Here's how the part is built. I have some questions about the finished solid (model axes, mm). A direction names the side the tool comes from. Give positions to 0.01 mm unless a question says otherwise; leave off trailing zeros. Write each loop counter-clockwise with the first axis right and the second up, starting at its lowest first coordinate (ties: lowest second). Pieces come first, ordered by that corner, then holes. Notation, with made-up numbers: (30, 50) - (51, 50) arc R22 cw to (51, 77) - close; hole circle Ø5 at (-21.75, 6). An arc over 180 degrees is marked (long way). Write each question's results on one line, items separated by ' | '. Start each with the question number.
Item 1: Will these pins go through, and if not, where does the flat tip stop? P1, Ø2.5, axis at x = -14, z = -15.5, coming from the -Y side; P2, Ø5.5, axis at x = 15, z = -16.5, coming from the -Y side; P3, Ø1.5, axis at x = 27, y = 1.5, coming from the +Z side; P4, Ø1.4, axis at x = 13.716, z = -13.716, coming from the +Y side.
Item 2: Suppose I cut it at A-A on x = 7.5. List the corners of the cut face in (y, z) for me.
Item 3: Suppose I cut it at B-B on y = 3.5. List the corners of the cut face in (x, z) for me (3 decimals), then the cut area to 3 significant figures.
Item 4: Suppose I cut it at D-D on x = -32. List the corners of the cut face in (y, z) for me, then the cut area to 3 significant figures.
Item 5: Which directions (+Z, -Z, +X, -X, +Y, -Y) give clear straight access to the entire face, cutting with the end or side of a thin tool? Please do faces 1 (the flat face through (19.05, 3, 25)), 2 (the flat face through (-11.43, 3, -14)), 3 (the flat face through (15, 0.508, -14)).
Item 6: Suppose I cut it at C-C on z = 22. List the corners of the cut face in (x, y) for me.
Item 7: Please list where these lines run through material, in increasing order: line 1 along Z through (x, y) = (3.5, 3.15); line 2 along X through (y, z) = (3.25, -17.5); line 3 along Z through (x, y) = (29, 0.65).
```python
from build123d import *

# Parameters (mm, degrees)
BOSS_EXTRUDE1_DEPTH = 5.08
SKETCH2_R           = 1.778
CUT_EXTRUDE1_DEPTH  = 55.120480412
SKETCH3_W           = 22.86
SKETCH3_H           = 12.192
CUT_EXTRUDE2_DEPTH  = 4.572
SKETCH4_W           = 33.02
SKETCH4_H           = 12.192
CUT_EXTRUDE3_DEPTH  = 0.508
SKETCH5_R           = 0.889
CUT_EXTRUDE4_DEPTH  = 55.075162358


with BuildPart() as part:
    # Sketch1 → Boss-Extrude1 (new body)
    with BuildSketch(Plane(origin=(0, 0, 0), x_dir=(1, 0, 0), z_dir=(0, 1, 0))):
        Polygon((-38.1, -12.7), (-38.1, 38.1), (38.1, 38.1), (38.1, -12.7), (19.05, -12.7), (19.05, -38.1), (-19.05, -38.1), (-19.05, -12.7), align=None)
    extrude(amount=BOSS_EXTRUDE1_DEPTH)

    # Sketch2 → Cut-Extrude1 (cut, through all)
    with BuildSketch(Plane(origin=(0, 5.08, 0), x_dir=(1, 0, 0), z_dir=(0, 1, 0))):
        with Locations(Location((-22.225, 29.972, 0), (0, 0, 270))):
            Circle(SKETCH2_R)
        with Locations(Location((22.225, 29.972, 0), (0, 0, 90))):
            Circle(SKETCH2_R)
    extrude(amount=-CUT_EXTRUDE1_DEPTH, mode=Mode.SUBTRACT)

    # Sketch3 → Cut-Extrude2 (cut)
    with BuildSketch(Plane(origin=(0, 5.08, 0), x_dir=(1, 0, 0), z_dir=(0, 1, 0))):
        with Locations((0, 13.716)):
            Rectangle(SKETCH3_W, SKETCH3_H)
    extrude(amount=-CUT_EXTRUDE2_DEPTH, mode=Mode.SUBTRACT)

    # Sketch4 → Cut-Extrude3 (cut)
    with BuildSketch(Plane.XZ):
        with Locations((0, -13.716)):
            Rectangle(SKETCH4_W, SKETCH4_H)
    extrude(amount=-CUT_EXTRUDE3_DEPTH, mode=Mode.SUBTRACT)

    # Sketch5 → Cut-Extrude4 (cut, through all)
    with BuildSketch(Plane.XZ.offset(-0.508)):
        with Locations(Location((-13.716, -13.716, 0), (0, 0, 270))):
            Circle(SKETCH5_R)
        with Locations(Location((13.716, -13.716, 0), (0, 0, 270))):
            Circle(SKETCH5_R)
    extrude(amount=-CUT_EXTRUDE4_DEPTH, mode=Mode.SUBTRACT)


solid = part.part
```
Checked values:
1) P1: stops at y = 0.51 | P2: stops at y = 0 | P3: stops at z = 12.7 | P4: passes through
2) outline: (0, -38.1) - (5.08, -38.1) - (5.08, -19.81) - (0, -19.81) - close; (0, -7.62) - (5.08, -7.62) - (5.08, 38.1) - (0, 38.1) - close
3) outline: (-38.1, -38.1) - (38.1, -38.1) - (38.1, 12.7) - (19.05, 12.7) - (19.05, 38.1) - (-19.05, 38.1) - (-19.05, 12.7) - (-38.1, 12.7) - close; hole circle Ø3.556 at (-22.225, -29.972); hole circle Ø1.778 at (-13.716, -13.716); hole (-11.43, -19.812) - (11.43, -19.812) - (11.43, -7.62) - (-11.43, -7.62) - close; hole circle Ø1.778 at (13.716, -13.716); hole circle Ø3.556 at (22.225, -29.972) | area: 4,540 mm^2
4) outline: (0, -38.1) - (5.08, -38.1) - (5.08, 12.7) - (0, 12.7) - close | area: 258 mm^2
5) face 1: +Z, +X, +Y, -Y | face 2: +Y, -Y | face 3: -Y
6) outline: (-19.05, 0) - (19.05, 0) - (19.05, 5.08) - (-19.05, 5.08) - close
7) line 1: z = -38.1 to -19.81, -7.62 to 38.1 | line 2: x = -38.1 to -11.43, 11.43 to 38.1 | line 3: z = -38.1 to 12.7
